Source: CAD feature listing. Evaluate the final solid. Frame: model axes, mm. A direction names the side the tool comes from. Coordinates: 2 decimals unless noted, no trailing zeros. Loops run counter-clockwise (first coordinate to the right, second up) from the corner with the lowest first, then second, coordinate; pieces in that order, holes last. Notation, with made-up numbers: (-17, 82) -> (11, 82) arc R11 cw to (11, 87) -> close; hole circle Ø7 at (-33.5, 5). An arc over 180 degrees is marked (long way). Answer as CSV lines item,"result".
from build123d import *

# Parameters (mm, degrees)
SKETCH2_R           = 30
BOSS_EXTRUDE1_DEPTH = 6.8
SKETCH3_R           = 13.25
SKETCH3_R_2         = 7.25
BOSS_EXTRUDE2_DEPTH = 4.7
FILLET1_R           = 15
SKETCH6_R           = 5.75
CUT_EXTRUDE3_DEPTH  = 4.7
CIRPATTERN1_COUNT   = 4
SKETCH7_R           = 7.25
CUT_EXTRUDE4_DEPTH  = 44.957365708


with BuildPart() as part:
    # Sketch2 → Boss-Extrude1 (new body)
    with BuildSketch(Plane(origin=(0, 0, 0), x_dir=(1, 0, 0), z_dir=(0, 1, 0))):
        with Locations(Location((0, 0, 0), (0, 0, 270))):
            Circle(SKETCH2_R)
    extrude(amount=BOSS_EXTRUDE1_DEPTH)

    # Sketch3 → Boss-Extrude2 (add)
    with BuildSketch(Plane(origin=(0, 6.8, 0), x_dir=(1, 0, 0), z_dir=(0, 1, 0))):
        with Locations(Location((0, 0, 0), (0, 0, 270))):
            Circle(SKETCH3_R)
        with Locations(Location((0, 0, 0), (0, 0, 270))):
            Circle(SKETCH3_R_2, mode=Mode.SUBTRACT)
    extrude(amount=BOSS_EXTRUDE2_DEPTH)

    # Fillet1
    # the kernel refuses this fillet: 15 mm, written as the material it adds along each edge
    with BuildSketch(Plane(origin=(0, 6.8, 0), x_dir=(0, 0, 1), z_dir=(-1, 0, 0))) as fillet1_piece_1:
        with BuildLine():
            CenterArc((24.154586191, 15), FILLET1_R, 223.366822413, 46.633177587)
            Line((13.25, 4.7), (13.031908276, 4.494))
            ThreePointArc((13.031908276, 4.494), (12.95, 2.35), (12.95, 0))
            Line((12.95, 0), (13.25, -0.3))
            Line((13.25, -0.3), (24.154586191, -0.3))
            Line((24.154586191, -0.3), (24.154586191, 0))
        make_face()
    revolve(axis=Axis((0, 6.8, 0), (0, 1, 0)))

    # Sketch9 → CSK for M5 Hex Socket Countersunk Cap Screw1 (revolve, cut)
    with BuildSketch(Plane(origin=(0, 6.8, -20), x_dir=(0, 0, 1), z_dir=(1, 0, 0))):
        Polygon((0, 0), (0, 6.8), (2.75, 6.8), (2.75, 2.85), (5.6, 0), align=None)
    csk_for_m5_hex_socket_countersunk_cap_sc = revolve(axis=Axis((0, 13.15, -20), (0, -1, 0)), mode=Mode.SUBTRACT)

    # Sketch6 → Cut-Extrude3 (cut)
    with BuildSketch(Plane(origin=(0, 11.5, 0), x_dir=(1, 0, 0), z_dir=(0, 1, 0))):
        with Locations((0, 20)):
            Circle(SKETCH6_R)
    cut_extrude3 = extrude(amount=-CUT_EXTRUDE3_DEPTH, mode=Mode.SUBTRACT)

    # CirPattern1: CSK for M5 Hex Socket Countersunk Cap Screw1, Cut-Extrude3 ×4 about axis
    cirpattern1_axis = Axis((0, 0, 0), (0, 1, 0))
    add([csk_for_m5_hex_socket_countersunk_cap_sc.rotate(cirpattern1_axis, i * 360 / CIRPATTERN1_COUNT) for i in range(1, CIRPATTERN1_COUNT)], mode=Mode.SUBTRACT)
    add([cut_extrude3.rotate(cirpattern1_axis, i * 360 / CIRPATTERN1_COUNT) for i in range(1, CIRPATTERN1_COUNT)], mode=Mode.SUBTRACT)

    # Sketch7 → Cut-Extrude4 (cut, through all)
    with BuildSketch(Plane(origin=(0, 11.5, 0), x_dir=(1, 0, 0), z_dir=(0, 1, 0))):
        with Locations(Location((0, 0, 0), (0, 0, 270))):
            Circle(SKETCH7_R)
    extrude(amount=-CUT_EXTRUDE4_DEPTH, mode=Mode.SUBTRACT)


solid = part.part
(1) Pin query (flat end, axial travel): pin 1 Ø2 at (x, y) = (-3.5, 3) entering from -Z; pin 2 Ø2 at (y, z) = (2.5, -12) entering from -X; pin 3 Ø5 at (x, z) = (-15.5, -13.5) entering from +Y. Return the tip coordinate at first contact, or that it passes through.
Computed values:
pin 1,"z = -29.9"
pin 2,"x = -27.91"
pin 3,"y = 8.1"
(2) Access query for faces 1 (the cylindrical face through (-0.121, 2.003, -22.747)), 2 (the flat face through (-22, 6.8, 11)). Directions: +Z, -Z, +X, -X, +Y, -Y. A direction counts if a zero-diameter tool reaches every point of the face in a straight line with its end or side. Return the directions, or none.
Computed values:
face 1,"+Y, -Y"
face 2,"+Y"
(3) Cut plane A-A (z = 0). Return the cut outline in (x, y), then the cut area to 3 significant figures.
Computed values:
outline,"(-30, 0) -> (-22.75, 0) -> (-22.75, 3.95) -> (-25.6, 6.8) -> (-30, 6.8) -> close; (-17.25, 0) -> (-7.25, 0) -> (-7.25, 11.5) -> (-13.25, 11.5) arc R15 cw to (-14.25, 10.54) -> (-14.25, 6.8) -> (-14.4, 6.8) -> (-17.25, 3.95) -> close; (7.25, 0) -> (17.25, 0) -> (17.25, 3.95) -> (14.4, 6.8) -> (14.25, 6.8) -> (14.25, 10.54) arc R15 cw to (13.25, 11.5) -> (7.25, 11.5) -> close; (22.75, 0) -> (30, 0) -> (30, 6.8) -> (25.6, 6.8) -> (22.75, 3.95) -> close"
area,"283 mm^2"
(4) Material intervals for L1, parallel to Y at x = 14.5, z = -23.5; L2, parallel to Z at x = -3.5, y = 4.5; L3, parallel to Z at x = -23, y = 6.25, sorted ascending. Write a range as [from, to].
Computed values:
L1,"[0, 6.8]"
L2,"[-29.8, -6.35], [6.35, 29.8]"
L3,"[-19.26, -4.06], [4.06, 19.26]"
(5) Cut plane C-C (y = 3.25). Return the cut outline in (x, z), then the cut area to 3 significant figures.
Computed values:
outline,"circle Ø60 at (0, 0); hole circle Ø5.5 at (-20, 0); hole circle Ø14.5 at (0, 0); hole circle Ø5.5 at (0, -20); hole circle Ø5.5 at (0, 20); hole circle Ø5.5 at (20, 0)"
area,"2,570 mm^2"
(6) Draft query along Z for faces 3 (the cylindrical face through (0.121, 2.003, 22.747)), 4 (the flat face through (-6, 0, 6)), 5 (the cylindrical face through (1.32, 3.35, -29.97)). Return one class per face: released by +Z, released by -Z, zero draft, split by the parting line, or undercut.
Computed values:
face 3,"undercut"
face 4,"zero draft"
face 5,"split by the parting line"
(7) Cut plane B-B (x = 0). Return the cut outline in (y, z).
Computed values:
outline,"(0, -30) -> (6.8, -30) -> (6.8, -25.6) -> (3.95, -22.75) -> (0, -22.75) -> close; (0, -17.25) -> (3.95, -17.25) -> (6.8, -14.4) -> (6.8, -14.25) -> (10.54, -14.25) arc R15 cw to (11.5, -13.25) -> (11.5, -7.25) -> (0, -7.25) -> close; (0, 7.25) -> (11.5, 7.25) -> (11.5, 13.25) arc R15 cw to (10.54, 14.25) -> (6.8, 14.25) -> (6.8, 14.4) -> (3.95, 17.25) -> (0, 17.25) -> close; (0, 22.75) -> (3.95, 22.75) -> (6.8, 25.6) -> (6.8, 30) -> (0, 30) -> close"
(8) Cut plane D-D (y = 9.25). Return the cut outline in (x, z), then the cut area to 3 significant figures.
Computed values:
outline,"(-15.52, -3.61) arc R15.94 ccw to (-3.61, -15.52) arc R5.75 cw to (3.61, -15.52) arc R15.94 ccw to (15.52, -3.61) arc R5.75 cw to (15.52, 3.61) arc R15.94 ccw to (3.61, 15.52) arc R5.75 cw to (-3.61, 15.52) arc R15.94 ccw to (-15.52, 3.61) arc R5.75 cw to start; hole circle Ø14.5 at (0, 0)"
area,"600 mm^2"
